The figure shows three views and two pictorial views of one solid part (mm, origin at its lowest corner). Answer the questions. A direction names the side the tool comes from. Give positions to 0.01 mm unless a question says otherwise; leave off trailing zeros. Order: outer loops, then holes, each group sorted by start corner. A loop starts at its lowest first (then second) coordinate and runs counter-clockwise, first axis right, second up. Notation, with made-up numbers: (-29, -36) - (18, -36) arc R7 ccw to (18, -31) - close; hole circle Ø7 at (21.5, 37). An arc over 180 degrees is marked (long way). Write item = value, one per line.
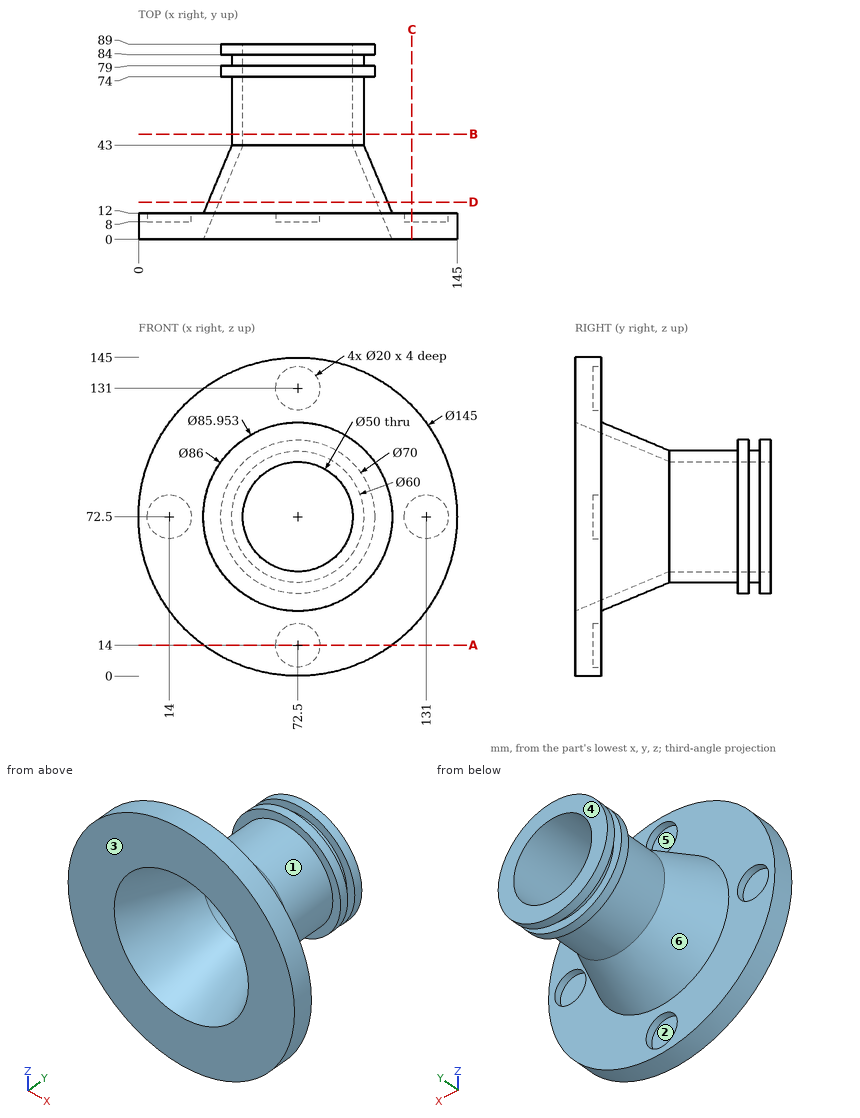
1. Section C-C (x = 124.5) is taken. Determine the outline of the cut face in (y, z), and give its area (3 significant figures).
Recorded:
outline = (0, 21.98) - (12, 21.98) - (12, 64.9) - (8, 64.9) - (8, 80.1) - (12, 80.1) - (12, 123.02) - (0, 123.02) - close
area = 1,150 mm^2
2. Determine the mould class of the marked faces 4, 5 and 6 for opening direction Z: +Z half, -Z half, draft (parallel to the pull), parting line (faces both ways), or undercut.
Recorded:
face_4 = draft
face_5 = undercut
face_6 = parting line
3. Section D-D (y = 17) is taken. Determine the outline of the cut face in (x, z).
Recorded:
outline = circle Ø81.77 at (72.5, 72.5); hole circle Ø71.77 at (72.5, 72.5)
4. Straight lines are drawn through the part: L1, parallel to X at y = 69, z = 72.5; L2, parallel to Z at x = 72, y = 76 (1 decimal). For each, find the intervals that lie inside material, in ascending order. Write a range as [from, to].
Recorded:
L1 = [42.5, 47.5], [97.5, 102.5]
L2 = [37.5, 47.5], [97.5, 107.5]
5. For the marked faces 1, 2 and 3, determine the directions among +Z, -Z, +X, -X, +Y, -Y from which every point of the face is accessible in a straight line to the end or side of a thin tool.
Recorded:
face_1 = none
face_2 = +Y
face_3 = +Z, -Z, +X, -X, -Y
6. Section A-A (z = 14) is taken. Determine the outline of the cut face in (x, y) (1 decimal).
Recorded:
outline = (29.7, 0) - (115.3, 0) - (115.3, 12) - (82.5, 12) - (82.5, 8) - (62.5, 8) - (62.5, 12) - (29.7, 12) - close
7. Flat-ended cylindrical pins translate along their axes: pin 1 (16 mm diameter, centred on x = 69, z = 131.5, fed in from +Y); pin 2 (8 mm diameter, centred on x = 93.5, y = 44, fed in from -Z) (1 decimal); pin 3 (18 mm diameter, centred on x = 72.5, z = 131, fed in from -Y); pin 4 (1.5 mm diameter, centred on x = 62, y = 44.5, fed in from -Z). Find the tip coordinate at first contact, or state that the pin passes through.
Recorded:
pin_1 = 12
pin_2 = 47.6
pin_3 = 0
pin_4 = 44.13
8. Section B-B (y = 48) is taken. Determine the outline of the cut face in (x, z).
Recorded:
outline = circle Ø60 at (72.5, 72.5); hole circle Ø50 at (72.5, 72.5)
